Check sheet for the drawn part. Datum: minimum x, y, z corner. Units: mm. A direction names the side the tool comes from. Give positions to 0.01 mm unless a question says otherwise; leave off trailing zeros. Write each loop counter-clockwise with the first axis right and the second up, starting at its lowest first coordinate (ties: lowest second). Pieces come first, ordered by that corner, then holes. Notation, with made-up numbers: (13, 3.25) - (24, 3.25) arc R27 cw to (24, 35.25) - close; hole circle Ø6 at (-7.5, -6). An arc over 180 degrees is marked (long way). Use a Markdown table: item, result.
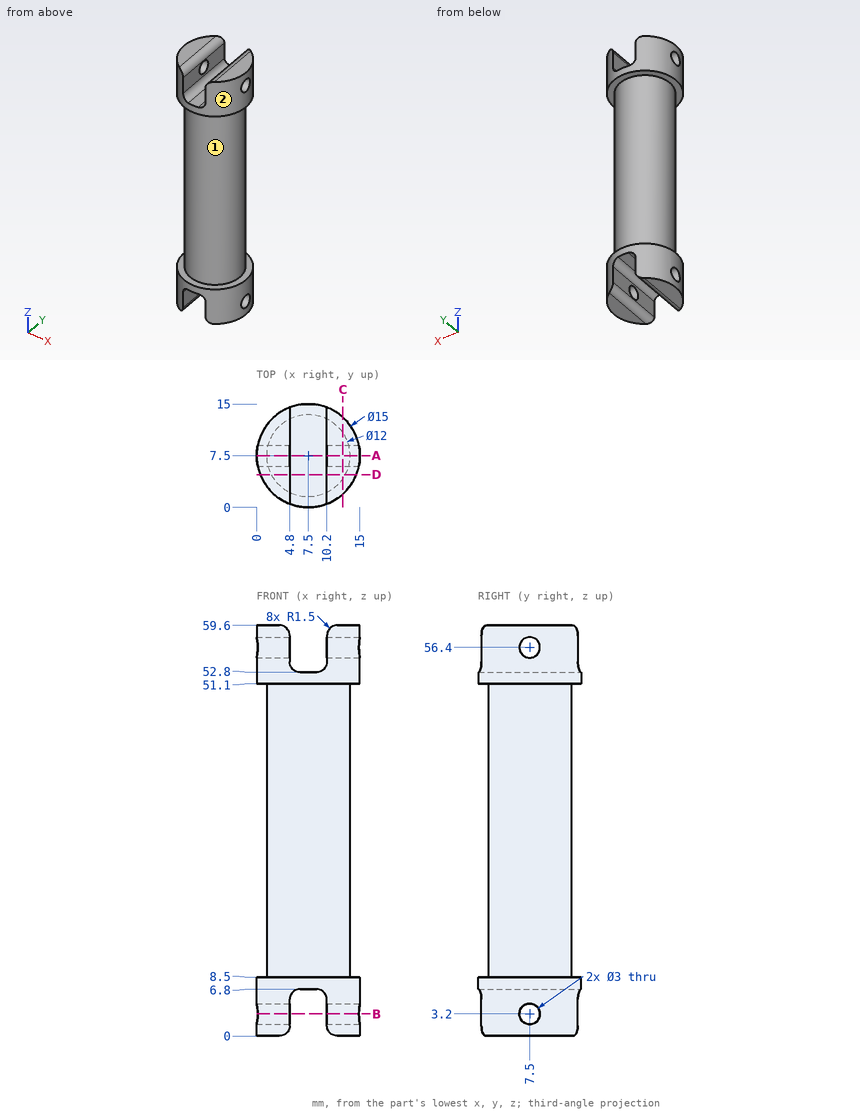
1) Material ranges on L1, parallel to Z at x = 2.75, y = 8.75; L2, parallel to Y at x = 7.5, z = 25; L3, parallel to Z at x = 4, y = 2.5, recorded low to high. Write a range as from..to.
Working result:
| item | result |
|---|---|
| L1 | z = 0..2.37, 4.03..55.57, 57.23..59.6 |
| L2 | y = 1.5..13.5 |
| L3 | z = 0.17..8.5, 51.1..59.43 |
2) Section check A-A on y = 7.5. Count the separate pieces of the cut face and the enclosed holes in it, then the cut area to 3 significant figures.
Working result:
| item | result |
|---|---|
| separate pieces | 5 |
| enclosed holes | 0 |
| area | 635 mm² |
3) Depth check by flat-ended pin: P1, Ø1, axis at x = 7, y = 6.5, coming from the -Z side; P2, Ø3, axis at x = 5.5, y = 13, coming from the +Z side; P3, Ø4, axis at x = 11.5, z = 36.5, coming from the -Y side. Enter the tip coordinate at first touch or a pass-through.
Working result:
| item | result |
|---|---|
| P1 | stops at z = 6.8 |
| P2 | stops at z = 59.43 |
| P3 | stops at y = 1.84 |
4) Section check B-B on z = 3.2. Record the boundary of the cut face in (x, y).
Working result:
| item | result |
|---|---|
| outline | (0.15, 6) arc R7.5 ccw to (4.8, 0.5) - (4.8, 6) - close; (0.15, 9) - (4.8, 9) - (4.8, 14.5) arc R7.5 ccw to start; (10.2, 0.5) arc R7.5 ccw to (14.85, 6) - (10.2, 6) - close; (10.2, 9) - (14.85, 9) arc R7.5 ccw to (10.2, 14.5) - close |
5) Set-up check for the marked faces 1 and 2: record each of +Z, -Z, +X, -X, +Y, -Y from which the full face is reachable in a straight line by a thin tool's end or side.
Working result:
| item | result |
|---|---|
| face 1 | none |
| face 2 | +Z, -Z |
6) Section check C-C on x = 12.5. Record the boundary of the cut face in (y, z).
Working result:
| item | result |
|---|---|
| outline | (1.91, 0) - (13.09, 0) - (13.09, 8.5) - (10.82, 8.5) - (10.82, 51.1) - (13.09, 51.1) - (13.09, 59.6) - (1.91, 59.6) - (1.91, 51.1) - (4.18, 51.1) - (4.18, 8.5) - (1.91, 8.5) - close; hole circle Ø3 at (7.5, 3.2); hole circle Ø3 at (7.5, 56.4) |
7) Section check D-D on y = 4.75. Record the boundary of the cut face in (x, z), then the cut area to 3 significant figures.
Working result:
| item | result |
|---|---|
| outline | (0.52, 0) - (3.3, 0) arc R1.5 ccw to (4.8, 1.5) - (4.8, 5.3) arc R1.5 cw to (6.3, 6.8) - (8.7, 6.8) arc R1.5 cw to (10.2, 5.3) - (10.2, 1.5) arc R1.5 ccw to (11.7, 0) - (14.48, 0) - (14.48, 8.5) - (12.83, 8.5) - (12.83, 51.1) - (14.48, 51.1) - (14.48, 59.6) - (11.7, 59.6) arc R1.5 ccw to (10.2, 58.1) - (10.2, 54.3) arc R1.5 cw to (8.7, 52.8) - (6.3, 52.8) arc R1.5 cw to (4.8, 54.3) - (4.8, 58.1) arc R1.5 ccw to (3.3, 59.6) - (0.52, 59.6) - (0.52, 51.1) - (2.17, 51.1) - (2.17, 8.5) - (0.52, 8.5) - close |
| area | 618 mm² |
